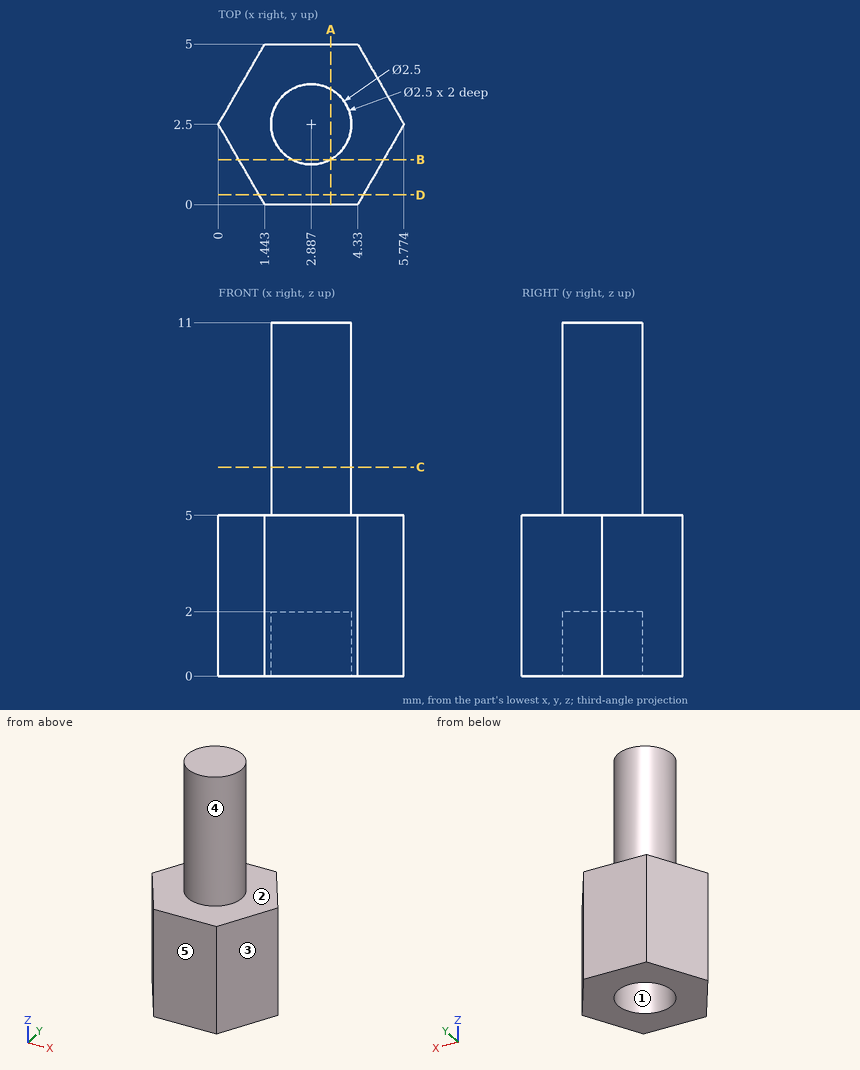
For this review, use the dimensioned drawing (mm, ordinates from the lowest corner) and the shaded views. A direction names the side the tool comes from. Coordinates: 2 decimals unless noted, no trailing zeros. Order: outer loops, then holes, each group sorted by start corner. A loop starts at its lowest first (then second) coordinate and runs counter-clockwise, first axis right, second up. Notation, with made-up numbers: M 86,75.5 L 98,75.5 A24 ccw 98,111.5 Z; hole C 38.25,64 d6. An arc over 180 degrees is marked long. Answer as a JSON object with one key per item and string values. Group by question number.
1) For pin 1 (2 mm diameter, centred on y = 0.5, z = 1.5, fed in from -X); pin 2 (1 mm diameter, centred on y = 0.5, z = 5, fed in from +X); pin 3 (2 mm diameter, centred on x = 5, y = 1, fed in from +Z), all flat-tipped, find the tip position at first contact; note any pin that passes through.
2) Add section B-B, the plane y = 1.4. Write out the cut boundary in (x, z) (1 decimal).
3) Add section A-A, the plane x = 3.5. Write out the cut boundary in (y, z), then the cut area to 3 significant figures.
4) Wall thickness on L1, parallel to Z at x = 1, y = 1.05; L2, parallel to Y at x = 2.4, z = 0.75; L3, parallel to Z at x = 2.95, y = 3.65: over which ranges is each line inside the solid? List them lowest first.
5) Mouldability with a two-part tool opening along Y and no side actions: class the marked faces 1, 2 and 3 as pulls with the +Y half, pulls with the -Y half, needs draft (parallel to the pull), parting line crosses it, or undercut.
6) Tool access review of the marked faces 4 and 5: name each direction out of +Z, -Z, +X, -X, +Y, -Y from which nothing blocks a thin tool from reaching the whole face with its end or side.
7) Add section D-D, the plane y = 0.3. Write out the cut boundary in (x, z), then the cut area to 3 significant figures.
8) Add section C-C, the plane z = 6.5. Write out the cut boundary in (x, y).
Computed values:
{
 "1": {"pin 1": "stops at x = 0.58", "pin 2": "stops at x = 4.91", "pin 3": "stops at z = 5"},
 "2": {"outline": "M 0.6,0 L 2.3,0 L 2.3,2 L 3.5,2 L 3.5,0 L 5.1,0 L 5.1,5 L 3.5,5 L 3.5,11 L 2.3,11 L 2.3,5 L 0.6,5 Z"},
 "3": {"outline": "M 0,0 L 1.41,0 L 1.41,2 L 3.59,2 L 3.59,0 L 5,0 L 5,5 L 3.59,5 L 3.59,11 L 1.41,11 L 1.41,5 L 0,5 Z", "area": "33.7 mm^2"},
 "4": {"L1": "z = 0 to 5", "L2": "y = 0 to 1.35, 3.65 to 5", "L3": "z = 2 to 11"},
 "5": {"face 1": "undercut", "face 2": "needs draft", "face 3": "pulls with the -Y half"},
 "6": {"face 4": "+Z", "face 5": "+Z, -Z, +X, -X, -Y"},
 "7": {"outline": "M 1.27,0 L 4.5,0 L 4.5,5 L 1.27,5 Z", "area": "16.2 mm^2"},
 "8": {"outline": "C 2.89,2.5 d2.5"}
}
